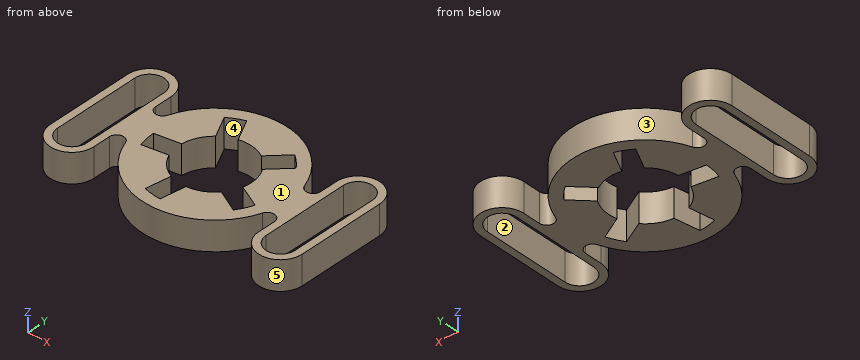
```python
from build123d import *

# Parameters (mm, degrees)
BOSS_EXTRUDE1_DEPTH = 10


with BuildPart() as part:
    # Sketch1 → Boss-Extrude1 (new, symmetric)
    with BuildSketch(Plane.XY):
        with BuildLine():
            Line((87, -30), (87, 30))
            ThreePointArc((87, 30), (72, 45), (57, 30))
            Line((57, 30), (57, 17.916472867))
            ThreePointArc((57, 17.916472867), (52.825722824, 12.985126011), (47.272727273, 16.287702607))
            ThreePointArc((47.272727273, 16.287702607), (0, 50), (-47.272727273, 16.287702607))
            ThreePointArc((-47.272727273, 16.287702607), (-52.825722824, 12.985126011), (-57, 17.916472867))
            Line((-57, 17.916472867), (-57, 30))
            ThreePointArc((-57, 30), (-72, 45), (-87, 30))
            Line((-87, 30), (-87, -30))
            ThreePointArc((-87, -30), (-72, -45), (-57, -30))
            Line((-57, -30), (-57, -17.916472867))
            ThreePointArc((-57, -17.916472867), (-52.825722824, -12.985126011), (-47.272727273, -16.287702607))
            ThreePointArc((-47.272727273, -16.287702607), (0, -50), (47.272727273, -16.287702607))
            ThreePointArc((47.272727273, -16.287702607), (52.825722824, -12.985126011), (57, -17.916472867))
            Line((57, -17.916472867), (57, -30))
            ThreePointArc((57, -30), (72, -45), (87, -30))
        make_face()
        with BuildLine():
            ThreePointArc((25.151236226, 33.636517601), (29.69848481, 29.69848481), (33.636517601, 25.151236226))
            Line((33.636517601, 25.151236226), (21.403642989, 12.918361615))
            ThreePointArc((21.403642989, 12.918361615), (24.084134557, 6.704808919), (25, 0))
            ThreePointArc((25, 0), (24.836482092, -2.85467289), (24.348067415, -5.672002568))
            Line((24.348067415, -5.672002568), (39.762388673, -13.525991536))
            ThreePointArc((39.762388673, -13.525991536), (37.422274016, -19.067600989), (34.314502676, -24.218069826))
            Line((34.314502676, -24.218069826), (18.900181419, -16.364080859))
            ThreePointArc((18.900181419, -16.364080859), (11.349762493, -22.275163105), (2.129571608, -24.90913336))
            Line((2.129571608, -24.90913336), (-0.576728553, -41.996040101))
            ThreePointArc((-0.576728553, -41.996040101), (-6.570247532, -41.482910305), (-12.42898864, -40.118826521))
            Line((-12.42898864, -40.118826521), (-9.722688479, -23.03191978))
            ThreePointArc((-9.722688479, -23.03191978), (-17.67766953, -17.67766953), (-23.03191978, -9.722688479))
            Line((-23.03191978, -9.722688479), (-40.118826521, -12.42898864))
            ThreePointArc((-40.118826521, -12.42898864), (-41.482910305, -6.570247532), (-41.996040101, -0.576728553))
            Line((-41.996040101, -0.576728553), (-24.90913336, 2.129571608))
            ThreePointArc((-24.90913336, 2.129571608), (-22.275163105, 11.349762493), (-16.364080859, 18.900181419))
            Line((-16.364080859, 18.900181419), (-24.218069826, 34.314502676))
            ThreePointArc((-24.218069826, 34.314502676), (-19.067600989, 37.422274016), (-13.525991536, 39.762388673))
            Line((-13.525991536, 39.762388673), (-5.672002568, 24.348067415))
            ThreePointArc((-5.672002568, 24.348067415), (3.910861626, 24.692208515), (12.918361615, 21.403642989))
            Line((12.918361615, 21.403642989), (25.151236226, 33.636517601))
        make_face(mode=Mode.SUBTRACT)
        with BuildLine():
            Line((-82, -30), (-82, 30))
            ThreePointArc((-82, 30), (-72, 40), (-62, 30))
            Line((-62, 30), (-62, -30))
            ThreePointArc((-62, -30), (-72, -40), (-82, -30))
        make_face(mode=Mode.SUBTRACT)
        with BuildLine():
            ThreePointArc((62, 30), (72, 40), (82, 30))
            Line((82, 30), (82, -30))
            ThreePointArc((82, -30), (72, -40), (62, -30))
            Line((62, -30), (62, 30))
        make_face(mode=Mode.SUBTRACT)
    extrude(amount=BOSS_EXTRUDE1_DEPTH, both=True)


solid = part.part
```
For this review, take the finished solid that the model builds, in its own axes (mm). Face numbers are marked on the shaded views. A direction names the side the tool comes from. Coordinates: 2 decimals unless noted, no trailing zeros. Loops run counter-clockwise (first coordinate to the right, second up) from the corner with the lowest first, then second, coordinate; pieces in that order, holes last.
1. For the marked faces 4 and 5, list the 3-axis set-ups (+Z, -Z, +X, -X, +Y, -Y) from which the entire face can be reached by the end or side of a thin tool; tool diameter is ignored.
2. Mouldability with a two-part tool opening along Y and no side actions: class the marked faces 1, 2 and 3 as +Y half, -Y half, draft (parallel to the pull), parting line (faces both ways), or undercut.
3. For line 1 (X direction, y = -1, z = 0.5); line 2 (X direction, y = 2.5, z = 4.25); line 3 (X direction, y = 14.5, z = -7), list the stretches that pass through material, from the lowest coordinate up.
4. Add section D-D, the plane z = -8. Count the separate pieces of the cut face and the enclosed holes in it, then the cut area to 3 significant figures.
5. Add section A-A, the plane y = -32. Give the boundary of the cut face in (x, z).
6. Add section B-B, the plane x = -68. Give the boundary of the cut face in (y, z).
7. Add section C-C, the plane y = -3.5. Give the boundary of the cut face in (x, z).
8. Insertion check: P1, Ø2, axis at y = 31.5, z = 3.5, coming from the +X side; P2, Ø6, axis at x = -64.5, z = -2, coming from the -Y side; P3, Ø12, axis at x = -13, z = -7, coming from the -Y side. Each pin has a flat end and moves straight along its axis. Give the tip position at first contact, or say it passes through.
Result:
1. face 4: +Z, -Z
1. face 5: +Z, -Z, -Y
2. face 1: draft
2. face 2: undercut
2. face 3: +Y half
3. line 1: x = -87 to -82, -62 to -41.99, 24.98 to 62, 82 to 87
3. line 2: x = -87 to -82, -62 to -24.87, 24.87 to 62, 82 to 87
3. line 3: x = -87 to -82, -62 to -55.65, -48.35 to -20.37, 22.99 to 48.35, 55.65 to 62, 82 to 87
4. separate pieces: 1
4. enclosed holes: 3
4. area: 7,270 mm2
5. outline: (-86.87, -10) - (-81.8, -10) - (-81.8, 10) - (-86.87, 10) - close; (-62.2, -10) - (-57.13, -10) - (-57.13, 10) - (-62.2, 10) - close; (-38.42, -10) - (-11.14, -10) - (-11.14, 10) - (-38.42, 10) - close; (1.01, -10) - (38.42, -10) - (38.42, 10) - (1.01, 10) - close; (57.13, -10) - (62.2, -10) - (62.2, 10) - (57.13, 10) - close; (81.8, -10) - (86.87, -10) - (86.87, 10) - (81.8, 10) - close
6. outline: (-44.46, -10) - (-39.17, -10) - (-39.17, 10) - (-44.46, 10) - close; (39.17, -10) - (44.46, -10) - (44.46, 10) - (39.17, 10) - close
7. outline: (-87, -10) - (-82, -10) - (-82, 10) - (-87, 10) - close; (-62, -10) - (-41.85, -10) - (-41.85, 10) - (-62, 10) - close; (24.75, -10) - (62, -10) - (62, 10) - (24.75, 10) - close; (82, -10) - (87, -10) - (87, 10) - (82, 10) - close
8. P1: stops at x = 86.99
8. P2: stops at y = -44.31
8. P3: stops at y = -49.51
